```python
from build123d import *

# Parameters (mm, degrees)
ESQUISSE1_R          = 13.375
ESQUISSE1_R_2        = 1.35
BASE_EXTRUSION_DEPTH = 0.75


with BuildPart() as part:
    # Esquisse1 → Base-Extrusion (new body)
    with BuildSketch(Plane.XY):
        with BuildLine():
            Line((-4.752719099, 14.490485194), (-11.490485194, 14.490485194))
            ThreePointArc((-11.490485194, 14.490485194), (-14.190687351, 12.797737393), (-13.843715332, 9.629757402))
            ThreePointArc((-13.843715332, 9.629757402), (-13.316796605, 8.324376183), (-13.578720666, 6.941242329))
            ThreePointArc((-13.578720666, 6.941242329), (-14.258481428, 5.409085631), (-14.765986011, 3.811581971))
            ThreePointArc((-14.765986011, 3.811581971), (-14.96384856, 2.940363289), (-15.110354082, 2.059053064))
            ThreePointArc((-15.110354082, 2.059053064), (-15.215048468, 1.031891528), (-15.25, 0))
            ThreePointArc((-15.25, 0), (-14.826294044, -3.569804606), (-13.578720666, -6.941242329))
            ThreePointArc((-13.578720666, -6.941242329), (-13.316796605, -8.324376183), (-13.843715332, -9.629757402))
            ThreePointArc((-13.843715332, -9.629757402), (-14.190687351, -12.797737393), (-11.490485194, -14.490485194))
            Line((-11.490485194, -14.490485194), (-4.752719099, -14.490485194))
            ThreePointArc((-4.752719099, -14.490485194), (0, -15.25), (4.752719099, -14.490485194))
            Line((4.752719099, -14.490485194), (11.490485194, -14.490485194))
            ThreePointArc((11.490485194, -14.490485194), (14.190687351, -12.797737393), (13.843715332, -9.629757402))
            ThreePointArc((13.843715332, -9.629757402), (13.316796605, -8.324376183), (13.578720666, -6.941242329))
            ThreePointArc((13.578720666, -6.941242329), (15.25, 0), (13.578720666, 6.941242329))
            ThreePointArc((13.578720666, 6.941242329), (13.316796605, 8.324376183), (13.843715332, 9.629757402))
            ThreePointArc((13.843715332, 9.629757402), (14.190687351, 12.797737393), (11.490485194, 14.490485194))
            Line((11.490485194, 14.490485194), (4.752719099, 14.490485194))
            ThreePointArc((4.752719099, 14.490485194), (2.406512081, 15.058924251), (0, 15.25))
            ThreePointArc((0, 15.25), (-2.406512081, 15.058924251), (-4.752719099, 14.490485194))
        make_face()
        Circle(ESQUISSE1_R, mode=Mode.SUBTRACT)
        with Locations((-11.490485194, -11.490485194)):
            Circle(ESQUISSE1_R_2, mode=Mode.SUBTRACT)
        with Locations((-11.490485194, 11.490485194)):
            Circle(ESQUISSE1_R_2, mode=Mode.SUBTRACT)
        with Locations((11.490485194, 11.490485194)):
            Circle(ESQUISSE1_R_2, mode=Mode.SUBTRACT)
        with Locations((11.490485194, -11.490485194)):
            Circle(ESQUISSE1_R_2, mode=Mode.SUBTRACT)
    extrude(amount=BASE_EXTRUSION_DEPTH)


solid = part.part
```
Source: CAD feature listing. Evaluate the final solid. Frame: model axes, mm. Give positions to 0.01 mm unless a question says otherwise; leave off trailing zeros. Loops run counter-clockwise (first coordinate to the right, second up) from the corner with the lowest first, then second, coordinate; pieces in that order, holes last. Notation, with made-up numbers: (-18, 9) -> (14, 9) arc R23 ccw to (14, 46) -> close; hole circle Ø1 at (82, 2). An arc over 180 degrees is marked (long way). Use a Markdown table: item, result. Add a question column.
(1) Ray query, line 1 (Y direction, x = -11, z = 0.3); line 2 (Y direction, x = -14, z = 0.2); line 3 (Y direction, x = -3.5, z = 0.1). Return the intervals inside material, ascending.
(2) Section query C-C (x = -9). Output: boundary loops of the cut face in (y, z).
(3) Section query B-B (z = 0.4). Output: boundary loops of the cut face in (x, y) (3 decimals).
(4) Pull-direction query (Y, two-part tool) for faces 1 (the face through (13, 4, 0)), 2 (the face through (-14.17, 12.84, 0.37)); classes: +Y half, -Y half, draft (parallel to the pull), parting line (faces both ways), or undercut.
(5) Section query A-A (y = 6). Output: boundary loops of the cut face in (x, z), then the cut area to 3 significant figures.
Checked values:
| question | item | result |
|---|---|---|
| 1 | line 1 | -14.49 to -12.75, -10.23 to -7.61, 7.61 to 10.23, 12.75 to 14.49 |
| 1 | line 2 | -13.13 to -9.85, -6.05 to 6.05, 9.85 to 13.13 |
| 1 | line 3 | -14.84 to -12.91, 12.91 to 14.84 |
| 2 | outline | (-14.49, 0) -> (-9.89, 0) -> (-9.89, 0.75) -> (-14.49, 0.75) -> close; (9.89, 0) -> (14.49, 0) -> (14.49, 0.75) -> (9.89, 0.75) -> close |
| 3 | outline | (-13.844, -9.63) arc R3 ccw to (-11.49, -14.49) -> (-4.753, -14.49) arc R15.25 ccw to (4.753, -14.49) -> (11.49, -14.49) arc R3 ccw to (13.844, -9.63) arc R2.5 cw to (13.579, -6.941) arc R15.25 ccw to (13.579, 6.941) arc R2.5 cw to (13.844, 9.63) arc R3 ccw to (11.49, 14.49) -> (4.753, 14.49) arc R15.25 ccw to (-4.753, 14.49) -> (-11.49, 14.49) arc R3 ccw to (-13.844, 9.63) arc R2.5 cw to (-13.579, 6.941) arc R15.25 ccw to (-13.579, -6.941) arc R2.5 cw to start; hole circle Ø26.75 at (0, 0); hole circle Ø2.7 at (-11.49, -11.49); hole circle Ø2.7 at (-11.49, 11.49); hole circle Ø2.7 at (11.49, -11.49); hole circle Ø2.7 at (11.49, 11.49) |
| 4 | face 1 | draft |
| 4 | face 2 | undercut |
| 5 | outline | (-14.02, 0) -> (-11.95, 0) -> (-11.95, 0.75) -> (-14.02, 0.75) -> close; (11.95, 0) -> (14.02, 0) -> (14.02, 0.75) -> (11.95, 0.75) -> close |
| 5 | area | 3.10 mm^2 |
